Can you work these out from the drawing? Everything is in mm from the part's minimum corner. Coordinates: 2 decimals unless noted, no trailing zeros. Order: outer loops, then holes, each group sorted by start corner. A loop starts at its lowest first (then second) coordinate and runs counter-clockwise, first axis right, second up. Notation, with made-up numbers: (-6.5, 53) -> (48.5, 53) arc R11 ccw to (48.5, 72) -> close; hole circle Ø3 at (-4.5, 28.5). An arc over 180 degrees is marked (long way). Write item = value, one per line. Start each with the question number.
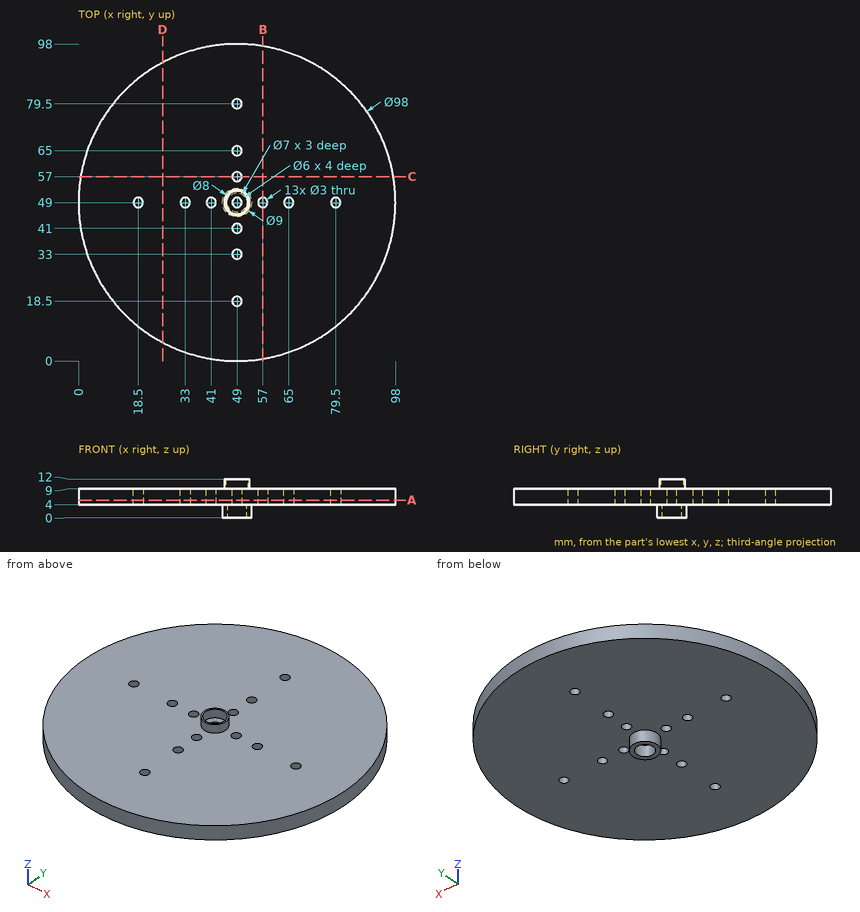
(1) Imagine slicing it at D-D (x = 26). Write out the boundary of the cut face in (y, z).
(2) Imagine slicing it at A-A (z = 5.5). Count the separate pieces of the cut face and the enclosed holes in it, plus the area to 3 significant figures.
(3) If I drill on L1, parallel to Y at x = 49, z = 1.2; L2, parallel to Z at x = 58, y = 78; L3, parallel to X at y = 6.5, z = 7, over which ranges is the centre line in solid material (lowest first)? Write a range as from..to.
(4) Imagine slicing it at B-B (x = 57). Write out the boundary of the cut face in (y, z).
(5) For P1, Ø2, axis at x = 48.5, y = 47.5, coming from the +Z side; P2, Ø4, axis at x = 23, y = 51.5, coming from the -Z side; P3, Ø5, axis at y = 69, z = 9.5, coming from the -X side, each with a flat end and sliding along its axis, tell me the tip position at first contact or that it passes through.
Result set:
q1.outline = (5.73, 4) -> (92.27, 4) -> (92.27, 9) -> (5.73, 9) -> close
q2.separate_pieces = 1
q2.enclosed_holes = 13
q2.area = 7,450 mm2
q3.L1 = 44.5..46, 52..53.5
q3.L2 = 4..9
q3.L3 = 24.61..73.39
q4.outline = (0.66, 4) -> (47.5, 4) -> (47.5, 9) -> (0.66, 9) -> close; (50.5, 4) -> (97.34, 4) -> (97.34, 9) -> (50.5, 9) -> close
q5.P1 = 9
q5.P2 = 4
q5.P3 = 3.25
